The model under review builds one solid part; all positions refer to its coordinate system, in mm. A direction names the side the tool comes from. Round coordinates to 2 decimals unless told otherwise and drop trailing zeros. Order: outer loops, then holes, each group sorted by start corner. A loop starts at its lowest first (then second) coordinate and runs counter-clockwise, first axis right, second up. Notation, with made-up numbers: M 45.5,-12 L 102.5,-12 A21 ccw 102.5,-5 Z; hole C 17,-10.5 d8. An arc over 180 degrees is marked long. Answer as a JSON object with one key per item and string values. Group by question number.
1. Add section A-A on x = 0. State the section outline as (y, z) points, and give its area (3 significant figures).
2. Add section B-B on z = 13.5. State the section outline as (x, y) points, and give its area (3 significant figures).
3. Mouldability with a two-part tool opening along Y and no side actions: class faces 4 (the face through (21, 1, 0)), 5 (the face through (21.33, -37.49, 6.22)), 6 (the face through (0, 38.5, 6)), 7 (the face through (0, -36.5, 6)) as released by +Y, released by -Y, zero draft, split by the parting line, or undercut.
4. Add section D-D on x = -26. State the section outline as (y, z) points, and give its area (3 significant figures).
5. To check wall thickness, follow probe 1 along X at (y, z) = (-9.5, 7); probe 2 along Z at (x, y) = (-21, 37); probe 3 along Y at (x, z) = (-15.5, 7). State the ranges of each line that lie inside material, in increasing order. Write a range as [from, to].
6. Machinability: for faces 1 (the face through (-0.81, -37.49, 9.06)), 2 (the face through (0, 36.5, 6)), 3 (the face through (-32.5, -1, 7)), which of the approach directions +Z, -Z, +X, -X, +Y, -Y give a long, thin tool a straight path to every point of the face, cutting with its end or side? Answer none if there is none.
7. Clearance check with flat-ended pins moving along their axes: P1, Ø4.5, axis at y = 0.5, z = 9, coming from the -X side; P2, Ø3, axis at y = -19, z = 10.5, coming from the +X side; P3, Ø9.5, axis at x = 21, y = 10, coming from the +Z side. State where each tip first meets the part, or that it passes through.
```python
from build123d import *

# Parameters (mm, degrees)
F0_W     = 65
F0_H     = 77
F0_W_2   = 2
F0_H_2   = 73
F1_DEPTH = 15
F3_DEPTH = 1.5
F5_R     = 1.5
F6_DEPTH = 80


with BuildPart() as f1:
    # F0 (on Top) → F1 (new body)
    with BuildSketch(Plane.XY):
        Rectangle(F0_W, F0_H)
        Polygon((11.5, 36.5), (30.5, 36.5), (30.5, -36.5), (11.5, -36.5), (9.5, -36.5), (-9.5, -36.5), (-11.5, -36.5), (-30.5, -36.5), (-30.5, 36.5), (-11.5, 36.5), (-9.5, 36.5), (9.5, 36.5), align=None, mode=Mode.SUBTRACT)
        with Locations((-10.5, 0)):
            Rectangle(F0_W_2, F0_H_2)
        with Locations((10.5, 0)):
            Rectangle(F0_W_2, F0_H_2)
    extrude(amount=F1_DEPTH)

    # F2 (on Top) → F3 (join)
    with BuildSketch(Plane.XY):
        Polygon((-32.663561, 37.936784), (-32.45391, -38.147267), (32.517858, -38.147267), (32.517858, 37.936784), align=None)
    extrude(amount=-F3_DEPTH)

    # F5 (on face) → F6 (cut)
    with BuildSketch(Plane(origin=(0, 38.5, 0), x_dir=(-1, 0, 0), z_dir=(0, 1, 0))):
        with Locations((-21, 7.682957)):
            Circle(F5_R)
        with Locations((0, 7.79829)):
            Circle(F5_R)
        with Locations((21, 7.682957)):
            Circle(F5_R)
    extrude(amount=-F6_DEPTH, mode=Mode.SUBTRACT)


solid = f1.part
```
Recorded:
{
 "1": {"outline": "M -38.5,0 L -38.15,0 L -38.15,-1.5 L 37.94,-1.5 L 37.94,0 L 38.5,0 L 38.5,6.3 L 36.5,6.3 L 36.5,0 L -36.5,0 L -36.5,6.3 L -38.5,6.3 Z; M -38.5,9.3 L -36.5,9.3 L -36.5,15 L -38.5,15 Z; M 36.5,9.3 L 38.5,9.3 L 38.5,15 L 36.5,15 Z", "area": "162 mm²"},
 "2": {"outline": "M -32.5,-38.5 L 32.5,-38.5 L 32.5,38.5 L -32.5,38.5 Z; hole M -30.5,-36.5 L -11.5,-36.5 L -11.5,36.5 L -30.5,36.5 Z; hole M -9.5,-36.5 L 9.5,-36.5 L 9.5,36.5 L -9.5,36.5 Z; hole M 11.5,-36.5 L 30.5,-36.5 L 30.5,36.5 L 11.5,36.5 Z", "area": "844 mm²"},
 "3": {"face 4": "undercut", "face 5": "zero draft", "face 6": "released by +Y", "face 7": "undercut"},
 "4": {"outline": "M -38.5,0 L -38.15,0 L -38.15,-1.5 L 37.94,-1.5 L 37.94,0 L 38.5,0 L 38.5,15 L 36.5,15 L 36.5,0 L -36.5,0 L -36.5,15 L -38.5,15 Z", "area": "174 mm²"},
 "5": {"probe 1": "x = [-32.5, -30.5], [-11.5, -9.5], [9.5, 11.5], [30.5, 32.5]", "probe 2": "z = [-1.5, 6.18], [9.18, 15]", "probe 3": "y = [-38.5, -36.5], [36.5, 38.5]"},
 "6": {"face 1": "+Y, -Y", "face 2": "+Z", "face 3": "+Z, -X, +Y, -Y"},
 "7": {"P1": "stops at x = -32.5", "P2": "stops at x = 32.5", "P3": "stops at z = 0"}
}
